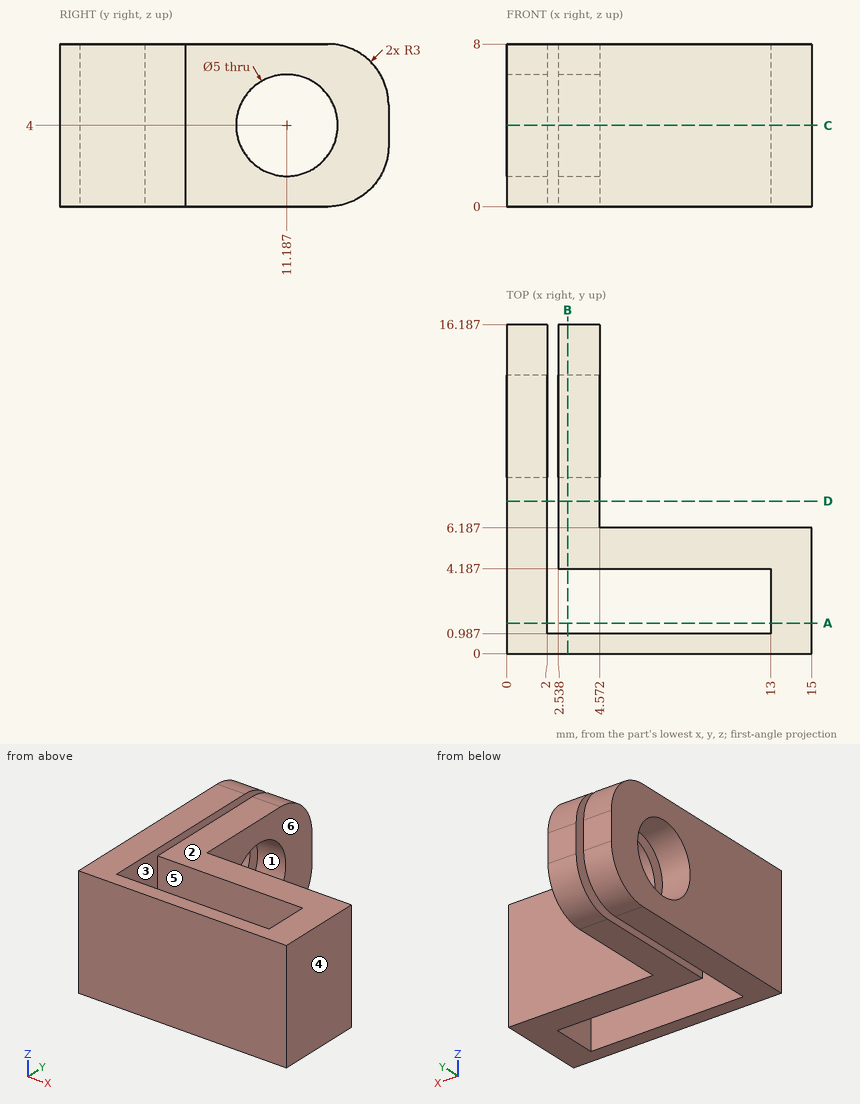
Drawing for the job (mm, zero at the part's lowest x, y, z). A direction names the side the tool comes from. Round coordinates to 2 decimals unless told otherwise and drop trailing zeros. Loops run counter-clockwise (first coordinate to the right, second up) from the corner with the lowest first, then second, coordinate; pieces in that order, holes last. Notation, with made-up numbers: (22.25, -36) - (81.25, -36) arc R20 ccw to (81.25, -27) - close; hole circle Ø11 at (43.25, 2.5). An arc over 180 degrees is marked (long way). Write each question's results on one line, items separated by ' | '.
(1) Saw through at D-D, the plane y = 7.5. List the corners of the cut face in (x, z).
Answer below:
outline: (0, 0) - (2, 0) - (2, 8) - (0, 8) - close; (2.54, 0) - (4.57, 0) - (4.57, 8) - (2.54, 8) - close
(2) Pin check, flat tips, straight feed: pin 1 (4 mm diameter, centred on y = 12, z = 6, fed in from +X); pin 2 (4.5 mm diameter, centred on y = 11.19, z = 4, fed in from -X); pin 3 (4 mm diameter, centred on x = 8, z = 4.5, fed in from +Y). Stop position of each tip, or through.
Answer below:
pin 1: stops at x = 4.57 | pin 2: passes through | pin 3: stops at y = 6.19
(3) Mould opens along Z. For the marked faces 1, 2 and 3 say: released by +Z, released by -Z, zero draft, split by the parting line, or undercut.
Answer below:
face 1: undercut | face 2: released by +Z | face 3: zero draft
(4) Saw through at A-A, the plane y = 1.5. List the corners of the cut face in (x, z).
Answer below:
outline: (0, 0) - (2, 0) - (2, 8) - (0, 8) - close; (13, 0) - (15, 0) - (15, 8) - (13, 8) - close
(5) Saw through at C-C, the plane z = 4. List the corners of the cut face in (x, y).
Answer below:
outline: (0, 0) - (15, 0) - (15, 6.19) - (4.57, 6.19) - (4.57, 8.69) - (2.54, 8.69) - (2.54, 4.19) - (13, 4.19) - (13, 0.99) - (2, 0.99) - (2, 8.69) - (0, 8.69) - close; (0, 13.69) - (2, 13.69) - (2, 16.19) - (0, 16.19) - close; (2.54, 13.69) - (4.57, 13.69) - (4.57, 16.19) - (2.54, 16.19) - close
(6) 3-axis set-ups, long thin cutter, end or side, ignore diameter. For the marked faces 4, 5 and 6: which of +Z, -Z, +X, -X, +Y, -Y reach the whole face in a straight line?
Answer below:
face 4: +Z, -Z, +X, +Y, -Y | face 5: +Z, -Z | face 6: +Z, -Z, +X, +Y
(7) Wall check: L1, parallel to X at y = 7.75, z = 3.5; L2, parallel to Y at x = 5.75, z = 2; L3, parallel to X at y = 5.25, z = 1. Give the ranges that are in metal, low to high.
Answer below:
L1: x = 0 to 2, 2.54 to 4.57 | L2: y = 0 to 0.99, 4.19 to 6.19 | L3: x = 0 to 2, 2.54 to 15
(8) Saw through at B-B, the plane x = 3. List the corners of the cut face in (y, z), then the cut area to 3 significant figures.
Answer below:
outline: (0, 0) - (0.99, 0) - (0.99, 8) - (0, 8) - close; (4.19, 0) - (13.19, 0) arc R3 ccw to (16.19, 3) - (16.19, 5) arc R3 ccw to (13.19, 8) - (4.19, 8) - close; hole circle Ø5 at (11.19, 4) | area: 80.4 mm^2
